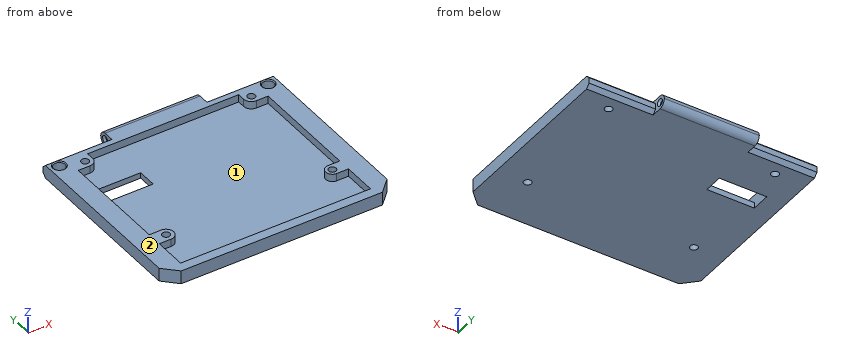
Autodesk Inventor part; units mm, degrees
ref_plane "YZ Plane" through (0, 0, 0) normal (1, 0, 0) x (0, 1, 0)
ref_plane "XZ Plane" through (0, 0, 0) normal (0, 1, 0) x (-1, 0, 0)
ref_plane "XY Plane" through (0, 0, 0) normal (0, 0, 1) x (1, 0, 0)
sketch "Sketch1" plane through (0, 0, 0) normal (0, 0, 1) x (1, 0, 0)
  line L0 (0, 100) -> (120, 100)
  line L1 (120, 100) -> (120, 0)
  line L2 (120, 0) -> (0, 0)
  line L3 (0, 0) -> (0, 100)
  line L4 (35, 100) -> (85, 100)
  line L5 (85, 100) -> (85, 107)
  line L6 (85, 107) -> (35, 107)
  line L7 (35, 107) -> (35, 100)
  point P0 (60, 100)
  dimension "d0" = 120
  dimension "d1" = 50
  dimension "d2" = 7
  dimension "d3" = 100
extrude "Extrusion1" add sketch "Sketch1" along normal blind 7
fillet "Fillet1" radius 3.5 2 edges at (60, 107, 7) (60, 107, 0)
sketch "Sketch2" plane through (85, 100, 7) normal (1, 0, 0) x (0, 0, -1)
  arc A0 (7, 3.5) -> (0, 3.5) centre (3.5, 3.5) ccw
  line L0 (0, 0) -> (0, 3.5)
  line L1 (7, 0) -> (0, 0)
  line L2 (7, 0) -> (7, 3.5)
  circle A1 centre (3.5, 3.5) radius 1
  point P0 (7, -100)
  dimension "d7" = 2
extrude "Extrusion2" cut sketch "Sketch2" against normal through all contours A1
ref_plane "Work Plane1" through (60, 0, 0) normal (1, 0, 0) x (0, 0, -1)
ref_plane "Work Plane2" through (0, 50, 0) normal (0, 1, 0) x (1, 0, 0)
chamfer "Chamfer1" distance 2 angle 45 4 edges at (17.5, 100, 7) (17.5, 100, 0) (102.5, 100, 0) (102.5, 100, 7)
sketch "Sketch3" plane through (0, 0, 7) normal (0, 0, 1) x (1, 0, 0)
  circle A0 centre (115, 94.5058) radius 3
  circle A1 centre (5, 94.5058) radius 3
  point P0 (0, 0)
extrude "Extrusion3" cut sketch "Sketch3" against normal blind 6
chamfer "Chamfer2" distance 0.5 angle 45 2 edges at (112, 94.5058, 7) (2, 94.5058, 7)
sketch "Sketch4" plane through (0, 0, 7) normal (0, 0, 1) x (1, 0, 0)
  line L0 (10, 95) -> (110, 95)
  line L1 (110, 95) -> (110, 5)
  line L2 (110, 5) -> (10, 5)
  line L3 (10, 5) -> (10, 95)
  line L4 (35, 100) -> (0, 100)
  line L5 (0, 98) -> (0, 0)
  line L6 (120, 0) -> (120, 98)
  line L7 (0, 0) -> (120, 0)
  line L8 (16.225, 91) -> (103.775, 91) construction
  line L9 (103.775, 91) -> (103.775, 26.1) construction
  line L10 (103.775, 26.1) -> (16.225, 26.1) construction
  line L11 (16.225, 26.1) -> (16.225, 91) construction
  circle A0 centre (16.225, 91) radius 4
  line L12 (20.225, 91) -> (20.225, 95)
  line L13 (16.225, 87) -> (10, 87)
  circle A1 centre (16.225, 26.1) radius 4
  line L14 (16.225, 30.1) -> (10, 30.1)
  line L15 (16.225, 22.1) -> (10, 22.1)
  circle A2 centre (103.775, 91) radius 4
  circle A3 centre (103.775, 26.1) radius 3.5
  line L16 (103.775, 29.6) -> (110, 29.6)
  line L17 (103.775, 22.6) -> (110, 22.6)
  line L18 (99.775, 91) -> (99.775, 95)
  line L19 (103.775, 87) -> (110, 87)
  point P0 (60, 91)
  point P1 (60, 95)
  dimension "d18" = 5
  dimension "d19" = 10
  dimension "d20" = 10
  dimension "d21" = 5
  dimension "d24" = 87.55
  dimension "d25" = 64.9
  dimension "d26" = 4
  dimension "d27" = 8
  dimension "d28" = 8
  dimension "d29" = 8
  dimension "d30" = 7
extrude "Extrusion4" cut sketch "Sketch4" against normal blind 4 contours L0 L18 A2 L19 L1 L16 A3 L17 L2 L3 L15 A1 L14 L13 A0 L12
sketch "Sketch5" plane through (0, 0, 7) normal (0, 0, 1) x (1, 0, 0)
  line L0 (103.775, 22.6) -> (110, 22.6)
  line L1 (110, 22.6) -> (110, 5)
  line L2 (110, 5) -> (10, 5)
  line L3 (10, 5) -> (10, 22.1)
  line L4 (10, 22.1) -> (16.225, 22.1)
  arc A0 (16.225, 22.1) -> (16.225, 30.1) centre (16.225, 26.1) ccw
  line L5 (16.225, 30.1) -> (10, 30.1)
  line L6 (10, 30.1) -> (10, 87)
  line L7 (10, 87) -> (16.225, 87)
  arc A1 (16.225, 87) -> (20.225, 91) centre (16.225, 91) ccw
  line L8 (20.225, 91) -> (20.225, 95)
  line L9 (20.225, 95) -> (99.775, 95)
  line L10 (99.775, 95) -> (99.775, 91)
  arc A2 (99.775, 91) -> (103.775, 87) centre (103.775, 91) ccw
  line L11 (103.775, 87) -> (110, 87)
  line L12 (110, 87) -> (110, 29.6)
  line L13 (110, 29.6) -> (103.775, 29.6)
  arc A3 (103.775, 29.6) -> (103.775, 22.6) centre (103.775, 26.1) ccw
  arc A4 (4.798, 98) -> (5.202, 98) centre (5, 94.5058) ccw
  line L14 (0, 98) -> (4.798, 98)
  line L15 (0, 98) -> (0, 0)
  line L16 (0, 0) -> (120, 0)
  line L17 (120, 0) -> (120, 98)
  line L18 (115.202, 98) -> (120, 98)
  arc A5 (114.798, 98) -> (115.202, 98) centre (115, 94.5058) ccw
  line L19 (85, 98) -> (114.798, 98)
  line L20 (85, 98) -> (85, 103.5)
  line L21 (35, 103.5) -> (85, 103.5)
  line L22 (35, 103.5) -> (35, 98)
  line L23 (5.202, 98) -> (35, 98)
hole "Hole1" at (16.225, 91, 7) at (16.225, 26.1, 7) at (103.775, 26.1, 7) at (103.775, 91, 7) direction (0, 0, -1) diameter 4 end through all
sketch "Sketch6" plane through (0, 0, 3) normal (0, 0, 1) x (1, 0, 0)
  line L0 (10, 30.1) -> (10, 87)
  line L1 (10, 75) -> (35, 75)
  line L2 (35, 75) -> (35, 65)
  line L3 (35, 65) -> (10, 65)
  line L4 (10, 65) -> (10, 75)
  line L5 (20.225, 95) -> (99.775, 95)
  point P0 (0, 0)
  point P1 (10, 65)
  dimension "d40" = 20
  dimension "d41" = 10
  dimension "d42" = 25
extrude "Extrusion5" cut sketch "Sketch6" against normal through all
chamfer "Chamfer3" distance 7 angle 45 2 edges at (120, 0, 3.5) (0, 0, 3.5)
chamfer "Chamfer4" distance 1 angle 45 2 edges at (35, 103.5, 4.5) (85, 103.5, 4.5)
properties part number "LCD Mount 2"
CAD build for the part. Positions are in the model's coordinates, mm. Face numbers are marked on the shaded views. Round coordinates to 2 decimals unless told otherwise and drop trailing zeros. Order: outer loops, then holes, each group sorted by start corner. A loop starts at its lowest first (then second) coordinate and runs counter-clockwise, first axis right, second up.
Q1. Slice it at A-A (x = 32). Write the cut outline in (y, z).
Q2. Wall check: L1, parallel to X at y = 26.1, z = 5 (3 decimals); L2, parallel to X at y = 91, z = 4.25 (3 decimals); L3, parallel to X at y = 43, z = 3.5. Give the ranges that are in metal, low to high.
Q3. Two-plate mould, pull along Y, no slides. Class the marked faces 1 and 2: pulls with the +Y half, pulls with the -Y half, needs draft (parallel to the pull), parting line crosses it, or undercut.
Q4. Slice it at C-C (y = 36). Write the cut outline in (x, z), and give its area (3 significant figures).
Q5. Drop flat-ended pins along their axis: pin 1 (2 mm diameter, centred on y = 102.5, z = 3, fed in from +X); pin 2 (1 mm diameter, centred on x = 18.5, z = 3, fed in from +Y); pin 3 (3 mm diameter, centred on x = 64.5, y = 35.5, fed in from +Z). Give the stop position or say it passes through.
Results below:
1. outline: (0, 0) - (65, 0) - (65, 3) - (5, 3) - (5, 7) - (0, 7) - close; (75, 0) - (98, 0) - (100, 2) - (100, 5) - (98, 7) - (95, 7) - (95, 3) - (75, 3) - close
2. L1: x = 0 to 14.225, 18.225 to 20.225, 100.275 to 101.775, 105.775 to 120
2. L2: x = 0 to 14.225, 18.225 to 20.225, 99.775 to 101.775, 105.775 to 120
2. L3: x = 0 to 10, 110 to 120
3. face 1: undercut
3. face 2: needs draft
4. outline: (0, 0) - (120, 0) - (120, 7) - (110, 7) - (110, 3) - (10, 3) - (10, 7) - (0, 7) - close
4. area: 440 mm2
5. pin 1: stops at x = 85
5. pin 2: stops at y = 100
5. pin 3: stops at z = 3
